```python
from build123d import *

# Parameters (mm, degrees)
BOSS_EXTRUDE1_DEPTH = 15
CUT_EXTRUDE1_REACH  = 41.051
SKETCH2_R           = 2
CUT_EXTRUDE2_REACH  = 38.069
SKETCH4_R           = 2
CUT_EXTRUDE3_DEPTH  = 15
SKETCH5_W           = 40
SKETCH5_H           = 4.1
CUT_EXTRUDE4_DEPTH  = 26
CUT_EXTRUDE6_REACH  = 39.299


with BuildPart() as part:
    # Sketch1 → Boss-Extrude1 (new body)
    with BuildSketch(Plane.XY):
        with BuildLine():
            Line((-20, 0), (20, 0))
            add(Edge.make_bspline(
                [(-20, 0), (-15, 30), (0, 40), (15, 30), (20, 0)],
                knots=[0, 0, 0, 0, 0, 1, 1, 1, 1, 1], degree=4))
        make_face()
    extrude(amount=BOSS_EXTRUDE1_DEPTH)

    # Sketch2 → Cut-Extrude1 (cut, up to next)
    with BuildSketch(Plane.XZ, mode=Mode.PRIVATE) as cut_extrude1_sk1:
        with Locations((16, 7.5)):
            Circle(SKETCH2_R)
    cut_extrude1_tool1 = extrude(cut_extrude1_sk1.sketch, amount=-CUT_EXTRUDE1_REACH, mode=Mode.PRIVATE) & part.part
    # Sketch2 → Cut-Extrude1 (cut, up to next)
    with BuildSketch(Plane.XZ, mode=Mode.PRIVATE) as cut_extrude1_sk2:
        with Locations((-16, 7.5)):
            Circle(SKETCH2_R)
    cut_extrude1_tool2 = extrude(cut_extrude1_sk2.sketch, amount=-CUT_EXTRUDE1_REACH, mode=Mode.PRIVATE) & part.part
    add(cut_extrude1_tool1.solids().sort_by_distance((16, 0, 7.5))[0], mode=Mode.SUBTRACT)
    add(cut_extrude1_tool2.solids().sort_by_distance((-16, 0, 7.5))[0], mode=Mode.SUBTRACT)

    # Sketch3 → Cut-Extrude2 (cut, up to next)
    with BuildSketch(Plane(origin=(0, 4, 0), x_dir=(-1, 0, 0), z_dir=(0, -1, 0)), mode=Mode.PRIVATE) as cut_extrude2_sk1:
        Polygon((17.732050808, -4.5), (14.267949192, -4.5), (12.535898385, -7.5), (14.267949192, -10.5), (17.732050808, -10.5), (19.464101615, -7.5), align=None)
    cut_extrude2_tool1 = extrude(cut_extrude2_sk1.sketch, amount=-CUT_EXTRUDE2_REACH, mode=Mode.PRIVATE) & part.part
    # Sketch3 → Cut-Extrude2 (cut, up to next)
    with BuildSketch(Plane(origin=(0, 4, 0), x_dir=(-1, 0, 0), z_dir=(0, -1, 0)), mode=Mode.PRIVATE) as cut_extrude2_sk2:
        Polygon((-17.732050808, -4.5), (-19.464101615, -7.5), (-17.732050808, -10.5), (-14.267949192, -10.5), (-12.535898385, -7.5), (-14.267949192, -4.5), align=None)
    cut_extrude2_tool2 = extrude(cut_extrude2_sk2.sketch, amount=-CUT_EXTRUDE2_REACH, mode=Mode.PRIVATE) & part.part
    add(cut_extrude2_tool1.solids().sort_by_distance((-16, 4, 7.5))[0], mode=Mode.SUBTRACT)
    add(cut_extrude2_tool2.solids().sort_by_distance((16, 4, 7.5))[0], mode=Mode.SUBTRACT)

    # Sketch4 → Cut-Extrude3 (cut)
    with BuildSketch(Plane.XY.offset(15)):
        with Locations((0, 10.25)):
            Circle(SKETCH4_R)
    extrude(amount=-CUT_EXTRUDE3_DEPTH, mode=Mode.SUBTRACT)

    # Sketch5 → Cut-Extrude4 (cut)
    with BuildSketch(Plane(origin=(0, 31, 0), x_dir=(1, 0, 0), z_dir=(0, 1, 0))):
        with Locations((0, -7.5)):
            Rectangle(SKETCH5_W, SKETCH5_H)
    extrude(amount=-CUT_EXTRUDE4_DEPTH, mode=Mode.SUBTRACT)

    # Cut-Extrude6: up to this face of the body (flat: up to its plane)
    cut_extrude6_end = Plane(part.part.faces().sort_by_distance((3.91e-07, 16.202361225, 5.45))[0])
    # Sketch7 → Cut-Extrude6 (cut, up to the picked face)
    with BuildSketch(Plane(origin=(0, 0, 9.55), x_dir=(-1, 0, 0), z_dir=(0, 0, -1)), mode=Mode.PRIVATE) as cut_extrude6_sk1:
        with BuildLine():
            Line((13.719466437, 5), (13.719466437, 6.244656836))
            Line((13.719466437, 6.244656836), (-13.719466437, 6.244656836))
            Line((-13.719466437, 6.244656836), (-13.719466437, 5))
            ThreePointArc((-13.719466437, 5), (0, 1.028956083), (13.719466437, 5))
        make_face()
    cut_extrude6_tool1 = split(extrude(cut_extrude6_sk1.sketch, amount=CUT_EXTRUDE6_REACH, mode=Mode.PRIVATE), bisect_by=cut_extrude6_end, keep=Keep.BOTH, mode=Mode.PRIVATE)
    add(cut_extrude6_tool1.solids().sort_by(Axis((0, 4.103163, 9.55), (0, 0, -1)))[0], mode=Mode.SUBTRACT)


solid = part.part
```
CAD build for the part. Positions are in the model's coordinates, mm. A direction names the side the tool comes from. Coordinates: 2 decimals unless noted, no trailing zeros. Return JSON: item names as keys, results as strings. Group by question number.
Q1. Flat gauge pins, fed straight in: pin 1 (0.8 mm diameter, centred on x = 19, z = 6, fed in from +Y); pin 2 (5 mm diameter, centred on x = -7, z = 7, fed in from +Y); pin 3 (1 mm diameter, centred on y = 11, z = 12.5, fed in from -X). Where does each tip first touch, or does it go through?
Q2. Cut at A-A, the plane x = 0. State how many separate pieces and enclosed holes the cut face has, then the cut area to 3 significant figures.
Q3. Drill centre lines: line 1 (Z direction, x = -16, y = 1.35); line 2 (Z direction, x = -4, y = 23); line 3 (Y direction, x = 0, z = 3.1). Where is each one in solid material? Low to high.
Q4. Pull direction Z, two halves, no side cores. Call faces 1 (the face through (13.855, 10.593, 9.785)), 2 (the face through (0, 16, 15)), 3 (the face through (0, 0, 7)): released by +Z, released by -Z, zero draft, split by the parting line, or undercut.
Q5. Which spindle directions (+Z, -Z, +X, -X, +Y, -Y) get a long thin tool onto all of the face, cutting with end or side? Do faces 4 (the face through (-17.474, 1.972, 8.852)), 5 (the face through (18.14, 6.24, 5.21)). Say none if no direction does.
Returned:
{
 "1": {"pin 1": "stops at y = 5", "pin 2": "stops at y = 28.76", "pin 3": "stops at x = -17.54"},
 "2": {"separate pieces": "3", "enclosed holes": "0", "area": "288 mm2"},
 "3": {"line 1": "z = 0 to 5.5, 9.5 to 15", "line 2": "z = 0 to 5.45, 9.55 to 15", "line 3": "y = 0 to 8.25, 12.25 to 30"},
 "4": {"face 1": "undercut", "face 2": "released by +Z", "face 3": "zero draft"},
 "5": {"face 4": "+Y, -Y", "face 5": "+Y"}
}
